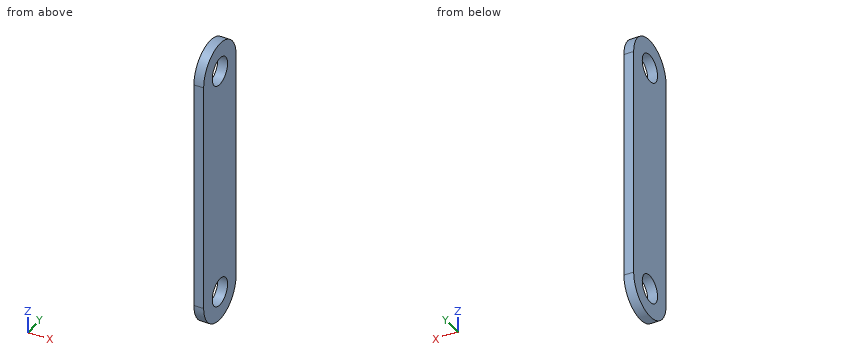
Autodesk Inventor part; units mm, degrees
ref_plane "YZ Plane" through (0, 0, 0) normal (1, 0, 0) x (0, 1, 0)
ref_plane "XZ Plane" through (0, 0, 0) normal (0, 1, 0) x (-1, 0, 0)
ref_plane "XY Plane" through (0, 0, 0) normal (0, 0, 1) x (1, 0, 0)
sketch "Sketch1" plane through (0, 0, 0) normal (1, 0, 0) x (0, 1, 0)
  circle A0 centre (0, 0) radius 2.2479
  circle A1 centre (0, -38.1) radius 2.2479
  arc A2 (4.7625, 0) -> (-4.7625, 0) centre (0, 0) ccw
  arc A3 (-4.7625, -38.1) -> (4.7625, -38.1) centre (0, -38.1) ccw
  line L0 (4.7625, 0) -> (4.7625, -38.1)
  line L1 (-4.7625, -38.1) -> (-4.7625, 0)
  dimension "d0" = 4.4958
  dimension "d1" = 4.4958
  dimension "d2" = 9.525
  dimension "d3" = 9.525
extrude "Extrusion1" add sketch "Sketch1" along normal blind 1.5875
properties part number "Motor Gearbox Gusset" material "Acetal Resin, White"
Can you work these out from the model? Positions are in its coordinate system, mm. Round coordinates to 2 decimals unless told otherwise and drop trailing zeros. Write each loop counter-clockwise with the first axis right and the second up, starting at its lowest first coordinate (ties: lowest second). Pieces come first, ordered by that corner, then holes. Notation, with made-up numbers: M -29.5,20 L 25.5,20 A31 cw 25.5,58 Z; hole C 7.25,71 d4. An arc over 180 degrees is marked long. Use a Markdown table: item, result.
Item 1: I want a section at B-B (z = 1). List the corners of the cut face in (x, y) for me.
Found:
| item | result |
|---|---|
| outline | M 0,-4.66 L 1.59,-4.66 L 1.59,-2.01 L 0,-2.01 Z; M 0,2.01 L 1.59,2.01 L 1.59,4.66 L 0,4.66 Z |
Item 2: If I drill on line 1 along Z through (x, y) = (0.5, 0); line 2 along Z through (x, y) = (1.3, 0.5); line 3 along Y through (x, z) = (1.3, -40), over which ranges is the centre line in solid material (lowest first)? Write a range as [from, to].
Found:
| item | result |
|---|---|
| line 1 | z = [-42.86, -40.35], [-35.85, -2.25], [2.25, 4.76] |
| line 2 | z = [-42.84, -40.29], [-35.91, -2.19], [2.19, 4.74] |
| line 3 | y = [-4.37, -1.2], [1.2, 4.37] |
Item 3: I want a section at A-A (y = 0). List the corners of the cut face in (x, z) for me.
Found:
| item | result |
|---|---|
| outline | M 0,-42.86 L 1.59,-42.86 L 1.59,-40.35 L 0,-40.35 Z; M 0,-35.85 L 1.59,-35.85 L 1.59,-2.25 L 0,-2.25 Z; M 0,2.25 L 1.59,2.25 L 1.59,4.76 L 0,4.76 Z |
Item 4: I want a section at C-C (x = 0.7). List the corners of the cut face in (y, z) for me (1 decimal).
Found:
| item | result |
|---|---|
| outline | M -4.8,-38.1 A4.8 ccw 4.8,-38.1 L 4.8,0 A4.8 ccw -4.8,0 Z; hole C 0,-38.1 d4.5; hole C 0,0 d4.5 |
